Here's how the part is built. I have some questions about the finished solid (model axes, mm). Coordinates: 2 decimals unless noted, no trailing zeros. Order: outer loops, then holes, each group sorted by start corner. A loop starts at its lowest first (then second) coordinate and runs counter-clockwise, first axis right, second up.
```python
from build123d import *

# Parameters (mm, degrees)
F0_R     = 0.5
F1_DEPTH = 0.25


with BuildPart() as f1:
    # F0 (on Top) → F1 (new body)
    with BuildSketch(Plane.XY):
        with BuildLine():
            Line((0.35, -2.3), (0.157627, -0.733249))
            ThreePointArc((0.157627, -0.733249), (0.749946, 0.008992), (0.14, 0.736817))
            Line((0.14, 0.736817), (0.14, 15.25))
            Line((0.14, 15.25), (0, 15.25))
            Line((0, 15.25), (-0.14, 15.25))
            Line((-0.14, 15.25), (-0.14, 0.736817))
            ThreePointArc((-0.14, 0.736817), (-0.749946, 0.008992), (-0.157627, -0.733249))
            Line((-0.157627, -0.733249), (-0.35, -2.3))
            Line((-0.35, -2.3), (0, -2.3))
            Line((0, -2.3), (0.35, -2.3))
        make_face()
        Circle(F0_R, mode=Mode.SUBTRACT)
    extrude(amount=F1_DEPTH)


solid = f1.part
```
Q1. If we section it at A-A on z = 0.1: Write out the boundary of the cut face in (x, y), then the cut area to 3 significant figures.
Q2. If we section it at C-C on y = 8.5: Write out the boundary of the cut face in (x, z).
Q3. If we section it at B-B on y = 0: Write out the boundary of the cut face in (x, z).
Q4. I need wall thicknesses on L1, parallel to Y at x = 0, z = 0.15; L2, parallel to X at y = 13.75, z = 0.15; L3, parallel to X at y = -0.25, z = 0.1. Which ranges of each line are inside material? Lowest first, please.
Reply:
1. outline: (-0.35, -2.3) - (0.35, -2.3) - (0.16, -0.73) arc R0.75 ccw to (0.14, 0.74) - (0.14, 15.25) - (-0.14, 15.25) - (-0.14, 0.74) arc R0.75 ccw to (-0.16, -0.73) - close; hole circle Ø1 at (0, 0)
1. area: 5.83 mm2
2. outline: (-0.14, 0) - (0.14, 0) - (0.14, 0.25) - (-0.14, 0.25) - close
3. outline: (-0.75, 0) - (-0.5, 0) - (-0.5, 0.25) - (-0.75, 0.25) - close; (0.5, 0) - (0.75, 0) - (0.75, 0.25) - (0.5, 0.25) - close
4. L1: y = -2.3 to -0.5, 0.5 to 15.25
4. L2: x = -0.14 to 0.14
4. L3: x = -0.71 to -0.43, 0.43 to 0.71
